Autodesk Inventor part; units mm, degrees
ref_plane "YZ Plane" through (0, 0, 0) normal (1, 0, 0) x (0, 1, 0)
ref_plane "XZ Plane" through (0, 0, 0) normal (0, 1, 0) x (-1, 0, 0)
ref_plane "XY Plane" through (0, 0, 0) normal (0, 0, 1) x (1, 0, 0)
sketch "Sketch1" plane through (0, 0, 0) normal (0, 1, 0) x (-1, 0, 0)
  circle A0 centre (-20.0808, -22.2584) radius 3.45
  circle A1 centre (-5.4083, -36.9307) radius 3.45
  line L0 (-25.35, -17) -> (-25.35, -23.6)
  line L1 (-25.35, -23.6) -> (-25.35, -35.6)
  line L2 (-25.35, -35.6) -> (-25.35, -42.2)
  line L3 (-25.35, -42.2) -> (-0.15, -42.2)
  line L4 (-0.15, -42.2) -> (-0.15, -35.6)
  line L5 (-0.15, -35.6) -> (-0.15, -23.6)
  line L6 (-0.15, -23.6) -> (-0.15, -17)
  line L7 (-25.35, -42.2) -> (-0.15, -42.2)
  line L8 (-0.15, -42.2) -> (-0.15, -17)
  line L9 (-0.15, -17) -> (-25.35, -17)
  line L10 (-25.35, -17) -> (-25.35, -42.2)
  circle A2 centre (-12.75, -29.6) radius 2.075
  point P0 (0, 0)
  point P1 (0, 0)
  dimension "d0" = 25.2
  dimension "d1" = 4.15
extrude "Extrusion1" add sketch "Sketch1" along normal blind 3
sketch "Sketch2" plane through (0, 0, 0) normal (0, -1, 0) x (1, 0, 0)
  point P0 (0, 0)
sketch "Sketch3" plane through (0, 0, 0) normal (0, -1, 0) x (1, 0, 0)
  circle A0 centre (12.75, -29.6) radius 2.075
  circle A1 centre (12.75, -29.6) radius 2.15
  point P0 (0, 0)
  dimension "d4" = 4.3
extrude "Extrusion2" cut sketch "Sketch3" against normal blind 10
sketch "Sketch4" plane through (0, 0, 0) normal (0, -1, 0) x (1, 0, 0)
  circle A0 centre (12.75, -29.6) radius 2.15
  circle A1 centre (12.75, -29.6) radius 2.35
  point P0 (0, 0)
  dimension "d7" = 4.7
extrude "Extrusion3" cut sketch "Sketch4" against normal blind 10
properties part number "upperSeal" material "Water"
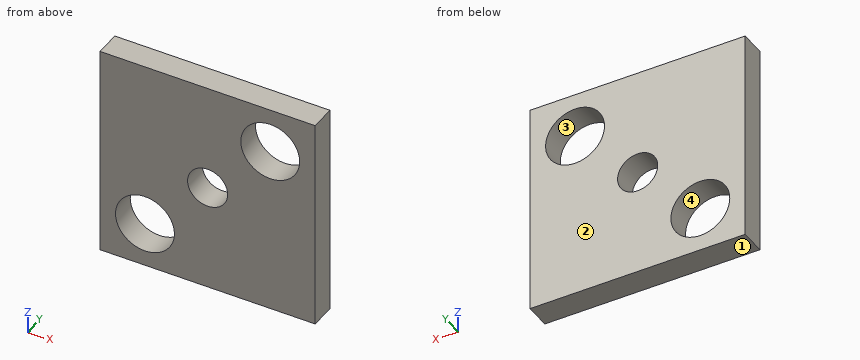
The model under review builds one solid part; all positions refer to its coordinate system, in mm. Face numbers are marked on the shaded views. Round coordinates to 2 decimals unless told otherwise and drop trailing zeros. Order: outer loops, then holes, each group sorted by start corner. A loop starts at its lowest first (then second) coordinate and runs counter-clockwise, first axis right, second up. Notation, with made-up numbers: (-17, -23) -> (-4, -23) arc R4 cw to (-4, -19) -> close; hole circle Ø6 at (57, -36.5). An arc over 180 degrees is marked (long way). Return JSON: item names as keys, results as strings.
1. For L1, parallel to Z at x = 12.75, y = 1.4; L2, parallel to X at y = 0.4, z = -37; L3, parallel to X at y = 2.65, z = -28, list the stretches that pass through material, from the lowest coordinate up. Write a range as [from, to].
Answer block:
{"L1": "z = [-42.2, -31.95], [-27.25, -17]", "L2": "x = [0.15, 1.96], [8.86, 25.35]", "L3": "x = [0.15, 11.03], [14.47, 25.35]"}
2. Take a section at B-B (x = 12.75). Write out the cut boundary in (y, z).
Answer block:
{"outline": "(0, -42.2) -> (3, -42.2) -> (3, -31.95) -> (0, -31.95) -> close; (0, -27.25) -> (3, -27.25) -> (3, -17) -> (0, -17) -> close"}
3. Take a section at A-A (z = -29.6). Write out the cut boundary in (x, y), then the cut area to 3 significant figures.
Answer block:
{"outline": "(0.15, 0) -> (10.4, 0) -> (10.4, 3) -> (0.15, 3) -> close; (15.1, 0) -> (25.35, 0) -> (25.35, 3) -> (15.1, 3) -> close", "area": "61.5 mm²"}
4. The part is to be moulded in two halves that separate along Z. For the marked faces 1, 2, 3 and 4, say which applies: +Z half, -Z half, draft (parallel to the pull), parting line (faces both ways), or undercut.
Answer block:
{"face 1": "-Z half", "face 2": "draft", "face 3": "undercut", "face 4": "undercut"}
5. Take a section at C-C (y = 1.05). Write out the cut boundary in (x, z), then the cut area to 3 significant figures.
Answer block:
{"outline": "(0.15, -42.2) -> (25.35, -42.2) -> (25.35, -17) -> (0.15, -17) -> close; hole circle Ø6.9 at (5.41, -36.93); hole circle Ø4.7 at (12.75, -29.6); hole circle Ø6.9 at (20.08, -22.26)", "area": "543 mm²"}
6. Insertion check: P1, Ø5.5, axis at x = 20.08, z = -22.26, coming from the +Y side. The pin has a flat end and moves straight along its axis. Give the tip position at first contact, or say it passes through.
Answer block:
{"P1": "passes through"}
